```python
from build123d import *

# Parameters (mm, degrees)
SKETCH1_W                                      = 124.8
SKETCH1_H                                      = 50.9
BOSS_EXTRUDE1_DEPTH                            = 1.45
CSK_FOR_M3_5_FLAT_HEAD_MACHINE_SCREW1_AT_COUNT = 2
CSK_FOR_M3_5_FLAT_HEAD_MACHINE_SCREW1_AT_PITCH = 115.5
CSK_FOR_M3_5_FLAT_HEAD_MACHINE_SCREW_2_COUNT   = 2
CSK_FOR_M3_5_FLAT_HEAD_MACHINE_SCREW_2_PITCH   = 123.420014584
CSK_FOR_M3_5_FLAT_HEAD_MACHINE_SCREW_3_COUNT   = 2
CSK_FOR_M3_5_FLAT_HEAD_MACHINE_SCREW_3_PITCH   = 43.5
FILLET2_R                                      = 4
SKETCH4_W                                      = 31.25
SKETCH4_H                                      = 11.25
CUT_EXTRUDE1_DEPTH                             = 1.45
FILLET3_R                                      = 0.5


with BuildPart() as part:
    # Sketch1 → Boss-Extrude1 (new body)
    with BuildSketch(Plane.XY):
        with Locations((62.4, -25.45)):
            Rectangle(SKETCH1_W, SKETCH1_H)
    extrude(amount=BOSS_EXTRUDE1_DEPTH)

    # Sketch2 → CSK for M3.5 Flat Head Machine Screw1 (revolve, cut)
    with BuildSketch(Plane(origin=(4.65, -3.7, 1.45), x_dir=(0, -1, 0), z_dir=(1, 0, 0))):
        Polygon((0, 0), (0, 1.45), (1.75, 1.45), (1.75, 1.294164458), (2.875, 0), align=None)
    csk_for_m3_5_flat_head_machine_screw1 = revolve(axis=Axis((4.65, -3.7, 7.8), (0, 0, -1)), mode=Mode.SUBTRACT)

    # CSK for M3.5 Flat Head Machine Screw1 at: CSK for M3.5 Flat Head Machine Screw1 ×2
    with Locations(*[(i * CSK_FOR_M3_5_FLAT_HEAD_MACHINE_SCREW1_AT_PITCH, 0, 0) for i in range(1, CSK_FOR_M3_5_FLAT_HEAD_MACHINE_SCREW1_AT_COUNT)]):
        add(csk_for_m3_5_flat_head_machine_screw1, mode=Mode.SUBTRACT)

    # CSK for M3.5 Flat Head Machine Screw 2: CSK for M3.5 Flat Head Machine Screw1 ×2
    with Locations(*[Vector(0.935828766, -0.35245499, 0) * (i * CSK_FOR_M3_5_FLAT_HEAD_MACHINE_SCREW_2_PITCH) for i in range(1, CSK_FOR_M3_5_FLAT_HEAD_MACHINE_SCREW_2_COUNT)]):
        add(csk_for_m3_5_flat_head_machine_screw1, mode=Mode.SUBTRACT)

    # CSK for M3.5 Flat Head Machine Screw 3: CSK for M3.5 Flat Head Machine Screw1 ×2
    with Locations(*[(0, -i * CSK_FOR_M3_5_FLAT_HEAD_MACHINE_SCREW_3_PITCH, 0) for i in range(1, CSK_FOR_M3_5_FLAT_HEAD_MACHINE_SCREW_3_COUNT)]):
        add(csk_for_m3_5_flat_head_machine_screw1, mode=Mode.SUBTRACT)

    # Fillet2
    fillet2_edges = [part.edges().sort_by_distance(p)[0] for p in [
        (0, 0, 0.725),
        (124.8, 0, 0.725),
        (124.8, -50.9, 0.725),
        (0, -50.9, 0.725),
    ]]
    fillet(fillet2_edges, radius=FILLET2_R)

    # Sketch4 → Cut-Extrude1 (cut)
    with BuildSketch(Plane.XY):
        with Locations((35.651, -10.75)):
            Rectangle(SKETCH4_W, SKETCH4_H)
        with Locations((89.651, -10.75)):
            Rectangle(SKETCH4_W, SKETCH4_H)
        with Locations((62.069, -40.5)):
            Rectangle(SKETCH4_W, SKETCH4_H)
    extrude(amount=CUT_EXTRUDE1_DEPTH, mode=Mode.SUBTRACT)

    # Fillet3
    fillet3_edges = [part.edges().sort_by_distance(p)[0] for p in [
        (77.694, -46.125, 0.725),
        (77.694, -34.875, 0.725),
        (46.444, -34.875, 0.725),
        (46.444, -46.125, 0.725),
        (105.276, -16.375, 0.725),
        (105.276, -5.125, 0.725),
        (74.026, -5.125, 0.725),
        (74.026, -16.375, 0.725),
        (51.276, -16.375, 0.725),
        (51.276, -5.125, 0.725),
        (20.026, -5.125, 0.725),
        (20.026, -16.375, 0.725),
    ]]
    fillet(fillet3_edges, radius=FILLET3_R)


solid = part.part
```
Work out the finished part from the listing and answer in its coordinate system (mm). Give positions to 0.01 mm unless a question says otherwise; leave off trailing zeros. Write each loop counter-clockwise with the first axis right and the second up, starting at its lowest first coordinate (ties: lowest second). Pieces come first, ordered by that corner, then holes. Notation, with made-up numbers: (18.5, 72.5) - (69.5, 72.5) arc R25 ccw to (69.5, 106.5) - close; hole circle Ø8 at (16, 78.5). An arc over 180 degrees is marked (long way). Use one line per item in the form item = value.
1. A cutting plane is placed at A-A (x = 26.5). Write down the section's boundary in (y, z) (3 decimals), and give its area (3 significant figures).
Filled in:
outline = (-50.9, 0) - (-16.375, 0) - (-16.375, 1.45) - (-50.9, 1.45) - close; (-5.125, 0) - (0, 0) - (0, 1.45) - (-5.125, 1.45) - close
area = 57.5 mm^2
2. Determine the mould class of faces 1 (the face through (123.597, -49.759, 0.735)), 2 (the face through (62, -25, 1.45)), 3 (the face through (123.597, -1.141, 0.735)) for opening direction Y: released by +Y, released by -Y, zero draft, split by the parting line, or undercut.
Filled in:
face_1 = released by -Y
face_2 = zero draft
face_3 = released by +Y
3. A cutting plane is placed at C-C (z = 0.9). State how many separate pieces and enclosed holes the cut face has, and give its area (3 significant figures).
Filled in:
separate_pieces = 1
enclosed_holes = 7
area = 5,210 mm^2
4. Consider L1, parallel to Y at x = 4.65, z = 0.1; L2, parallel to X at y = -3.7, z = 0.15; L3, parallel to X at y = -12, z = 0.7. Determine where each line is inside the solid, lowest interval first.
Filled in:
L1 = -50.9 to -48.95, -45.45 to -5.45, -1.95 to 0
L2 = 0.01 to 2.9, 6.4 to 118.4, 121.9 to 124.79
L3 = 0 to 20.03, 51.28 to 74.03, 105.28 to 124.8
5. A cutting plane is placed at B-B (y = -38). Write down the section's boundary in (x, z).
Filled in:
outline = (0, 0) - (46.44, 0) - (46.44, 1.45) - (0, 1.45) - close; (77.69, 0) - (124.8, 0) - (124.8, 1.45) - (77.69, 1.45) - close
